Can you work these out from the model? Positions are in its coordinate system, mm. Face numbers are marked on the shaded views. A direction names the side the tool comes from. Give positions to 0.01 mm unless a question says otherwise; leave off trailing zeros. Order: outer loops, then holes, each group sorted by start corner. A loop starts at its lowest first (then second) coordinate and runs counter-clockwise, first axis right, second up. Notation, with made-up numbers: (3, -9.5) - (23, -9.5) arc R18 ccw to (23, -0.5) - close; hole circle Ø10 at (71.25, 84). An arc over 180 degrees is marked (long way). Return JSON: item names as keys, results as strings.
Autodesk Inventor part; units mm, degrees
ref_plane "YZ Plane" through (0, 0, 0) normal (1, 0, 0) x (0, 1, 0)
ref_plane "XZ Plane" through (0, 0, 0) normal (0, 1, 0) x (-1, 0, 0)
ref_plane "XY Plane" through (0, 0, 0) normal (0, 0, 1) x (1, 0, 0)
sketch "Sketch1" plane through (0, 0, 0) normal (1, 0, 0) x (0, 1, 0)
  point P0 (0, 0)
sketch "Sketch2" plane through (0, 0, 0) normal (1, 0, 0) x (0, 1, 0)
  circle A0 centre (0, 0) radius 18.4
  dimension "d0" = 36.8
extrude "Extrusion1" add sketch "Sketch2" along normal blind 22
sketch "Sketch3" plane through (22, 0, 0) normal (1, 0, 0) x (0, 0, -1)
  line L0 (0, 0) -> (0, -7)
  circle A0 centre (0, -7) radius 6
  dimension "d3" = 7
  dimension "d4" = 12
extrude "Extrusion2" add sketch "Sketch3" along normal blind 6.4
chamfer "Chamfer1" distance 1 angle 45 1 edges at (28.4, -7, 6)
sketch "Sketch4" plane through (28.4, -7, 0) normal (1, 0, 0) x (0, 0, -1)
  circle A0 centre (0, 0) radius 5
  circle A1 centre (0, 0) radius 3
  point P0 (0, 7)
  dimension "d10" = 6
extrude "Extrusion3" add sketch "Sketch4" along normal blind 12.5 contours A1
sketch "Sketch5" plane through (40.9, -7, 0) normal (1, 0, 0) x (0, 0, -1)
  circle A0 centre (0, 0) radius 3
  line L0 (0, -3) -> (0, 2.4)
  line L1 (0, 2.4) -> (1.8, 2.4)
  line L2 (-1.8, 2.4) -> (0, 2.4)
  point P0 (0, 7)
  dimension "d13" = 5.4
extrude "Extrusion4" cut sketch "Sketch5" against normal blind 12 contours L1 L2 A0
sketch "Sketch6" plane through (0, 0, 0) normal (-1, 0, 0) x (0, 0, 1)
  circle A0 centre (0, 0) radius 17.9
  dimension "d16" = 35.8
extrude "Extrusion5" add sketch "Sketch6" along normal blind 30
sketch "Sketch9" plane through (22, 0, 0) normal (1, 0, 0) x (0, 0, -1)
  circle A0 centre (0, 0) radius 15.5
  circle A1 centre (0, 15.5) radius 1.5
  circle A2 centre (15.5, 0) radius 1.5
  circle A3 centre (-15.5, 0) radius 1.5
  dimension "d19" = 31
  dimension "d20" = 3
  dimension "d21" = 3
  dimension "d22" = 3
extrude "Extrusion6" cut sketch "Sketch9" against normal blind 3 contours A0 A2 | A0 A2 | A1 A0 | A0 A1 | A3 A0 | A0 A3
properties part number "motor"
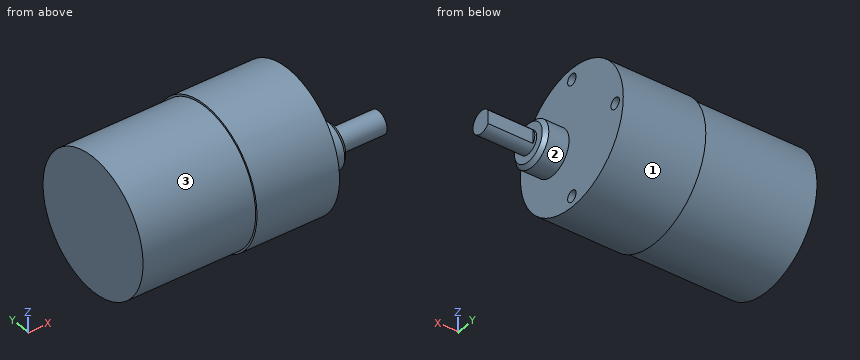
1. If I drill on L1, parallel to Z at x = 20, y = 0; L2, parallel to X at y = 16.5, z = -6; L3, parallel to Y at x = 20.65, z = 15.5, over which ranges is the centre line in solid material (lowest first)? Write a range as [from, to].
Checks:
{"L1": "[-18.4, -17], [-14, 14], [17, 18.4]", "L2": "[-30, 22]", "L3": "[-9.92, -1.5], [1.5, 9.92]"}
2. Suppose I cut it at B-B (z = 0). List the corners of the cut face in (x, y) for me.
Checks:
{"outline": "(-30, -17.9) - (0, -17.9) - (0, -18.4) - (22, -18.4) - (22, -13) - (27.4, -13) - (28.4, -12) - (28.4, -10) - (40.9, -10) - (40.9, -4.6) - (28.9, -4.6) - (28.9, -4) - (28.4, -4) - (28.4, -2) - (27.4, -1) - (22, -1) - (22, 14) - (19, 14) - (19, 17) - (22, 17) - (22, 18.4) - (0, 18.4) - (0, 17.9) - (-30, 17.9) - close"}
3. On a 3-axis mill with a long thin cutter (end or side, diameter ignored), from which of +Z, -Z, +X, -X, +Y, -Y can I reach the whole of each face in a straight line? I mean the marked faces 1, 2 and 3. Say none if no direction works.
Checks:
{"face 1": "+X, -X", "face 2": "+X", "face 3": "-X"}
4. For pin 1 Ø3.5 at (y, z) = (0.5, -15) entering from +X; pin 2 Ø8 at (x, y) = (19, -13) entering from -Z; pin 3 Ø1.5 at (y, z) = (0, 16) entering from +X; pin 4 Ø4 at (x, z) = (28.5, -8) entering from -Y, each with a flat end and sliding along its axis, tell me the tip position at first contact or that it passes through.
Checks:
{"pin 1": "x = 22", "pin 2": "z = -16.05", "pin 3": "x = 19", "pin 4": "through"}
5. Suppose I cut it at D-D (z = -15.5). List the corners of the cut face in (x, y) for me.
Checks:
{"outline": "(-30, -8.95) - (0, -8.95) - (0, -9.92) - (22, -9.92) - (22, -1.5) - (19, -1.5) - (19, 1.5) - (22, 1.5) - (22, 9.92) - (0, 9.92) - (0, 8.95) - (-30, 8.95) - close"}
6. Suppose I cut it at A-A (y = 0). List the corners of the cut face in (x, z) for me.
Checks:
{"outline": "(-30, -17.9) - (0, -17.9) - (0, -18.4) - (22, -18.4) - (22, -17) - (19, -17) - (19, -14) - (22, -14) - (22, 14) - (19, 14) - (19, 17) - (22, 17) - (22, 18.4) - (0, 18.4) - (0, 17.9) - (-30, 17.9) - close"}
7. Suppose I cut it at C-C (x = -6). List the corners of the cut face in (y, z) for me.
Checks:
{"outline": "circle Ø35.8 at (0, 0)"}
